Can you work these out from the drawing? Everything is in mm from the part's minimum corner. Round coordinates to 2 decimals unless told otherwise and drop trailing zeros. Loops run counter-clockwise (first coordinate to the right, second up) from the corner with the lowest first, then second, coordinate; pieces in that order, holes last. Notation, with made-up numbers: (66, 55.5) -> (118, 55.5) arc R32 cw to (118, 88.5) -> close; hole circle Ø2 at (64.5, -14.75). An arc over 180 degrees is marked (long way). Answer as a JSON object with one key per item and string values.
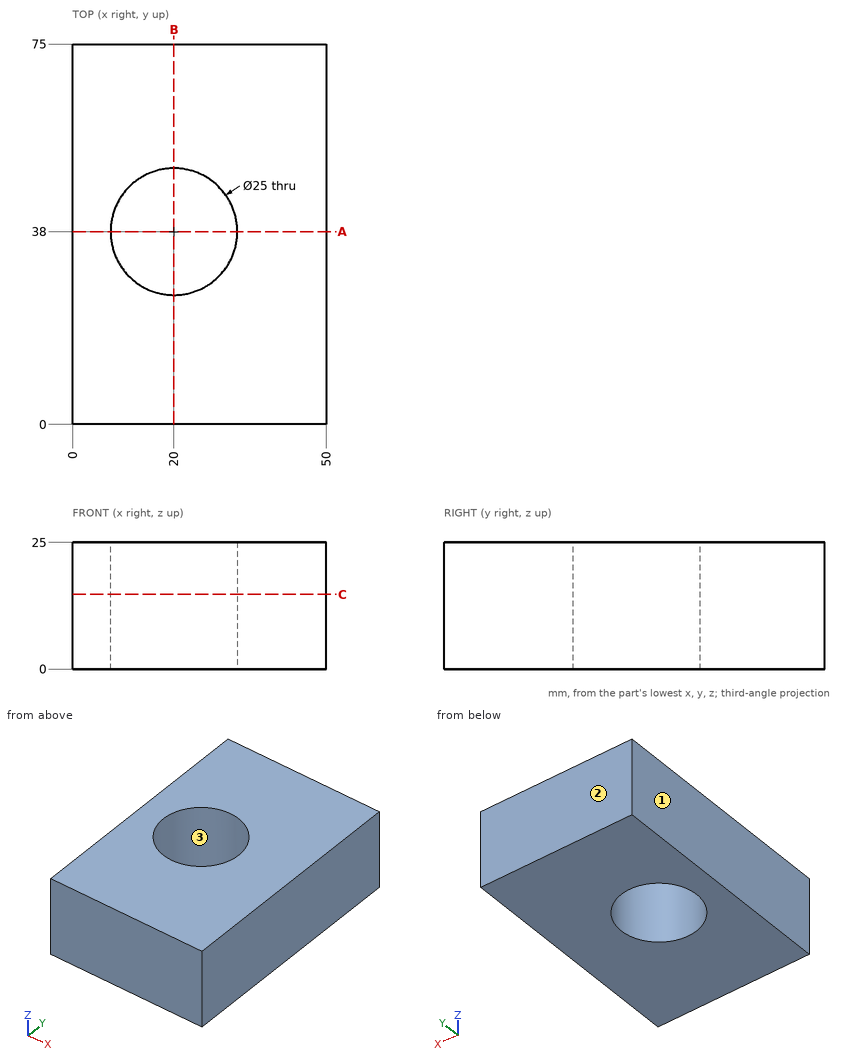
Q1. I want a section at B-B, the plane x = 20. Write out the boundary of the cut face in (y, z).
Determined:
{"outline": "(0, 0) -> (25.5, 0) -> (25.5, 25) -> (0, 25) -> close; (50.5, 0) -> (75, 0) -> (75, 25) -> (50.5, 25) -> close"}
Q2. If I drill on L1, parallel to Y at x = 20, z = 16; L2, parallel to X at y = 42, z = 10.75; L3, parallel to Y at x = 13, z = 13.25, over which ranges is the centre line in solid material (lowest first)? Write a range as [from, to].
Determined:
{"L1": "[0, 25.5], [50.5, 75]", "L2": "[0, 8.16], [31.84, 50]", "L3": "[0, 27.64], [48.36, 75]"}
Q3. I want a section at A-A, the plane y = 38. Write out the boundary of the cut face in (x, z), then the cut area to 3 significant figures.
Determined:
{"outline": "(0, 0) -> (7.5, 0) -> (7.5, 25) -> (0, 25) -> close; (32.5, 0) -> (50, 0) -> (50, 25) -> (32.5, 25) -> close", "area": "625 mm²"}
Q4. We'd pull the mould along Y, two halves only. Please class the marked faces 1, 2 and 3: pulls with the +Y half, pulls with the -Y half, needs draft (parallel to the pull), parting line crosses it, or undercut.
Determined:
{"face 1": "needs draft", "face 2": "pulls with the +Y half", "face 3": "undercut"}
Q5. I want a section at C-C, the plane z = 14.75. Write out the boundary of the cut face in (x, y), then the cut area to 3 significant figures.
Determined:
{"outline": "(0, 0) -> (50, 0) -> (50, 75) -> (0, 75) -> close; hole circle Ø25 at (20, 38)", "area": "3,260 mm²"}
